```python
from build123d import *

# Parameters (mm, degrees)
SKETCH_1_R      = 2
EXTRUDE_1_DEPTH = 250


with BuildPart() as part:
    # 草图1 → 凸台-拉伸1 (new, symmetric)
    with BuildSketch(Plane.XY):
        with BuildLine():
            Line((-8.5, 0), (-3.95, 0))
            ThreePointArc((-3.95, 0), (-3.737867966, 0.087867966), (-3.65, 0.3))
            Line((-3.65, 0.3), (-3.65, 0.6))
            Line((-3.65, 0.6), (-3.1, 0.6))
            Line((-3.1, 0.6), (-3.1, 1.8))
            Line((-3.1, 1.8), (-5.6, 1.8))
            Line((-5.6, 1.8), (-5.6, 3.692893219))
            Line((-5.6, 3.692893219), (-3.192893219, 6.1))
            Line((-3.192893219, 6.1), (3.192893219, 6.1))
            Line((3.192893219, 6.1), (5.6, 3.692893219))
            Line((5.6, 3.692893219), (5.6, 1.8))
            Line((5.6, 1.8), (3.1, 1.8))
            Line((3.1, 1.8), (3.1, 0.6))
            Line((3.1, 0.6), (3.65, 0.6))
            Line((3.65, 0.6), (3.65, 0.3))
            ThreePointArc((3.65, 0.3), (3.737867966, 0.087867966), (3.95, 0))
            Line((3.95, 0), (8.5, 0))
            ThreePointArc((8.5, 0), (9.560660172, 0.439339828), (10, 1.5))
            Line((10, 1.5), (10, 8.5))
            ThreePointArc((10, 8.5), (9.560660172, 9.560660172), (8.5, 10))
            Line((8.5, 10), (-8.5, 10))
            ThreePointArc((-8.5, 10), (-9.560660172, 9.560660172), (-10, 8.5))
            Line((-10, 8.5), (-10, 1.5))
            ThreePointArc((-10, 1.5), (-9.560660172, 0.439339828), (-8.5, 0))
        make_face()
        with Locations((-7, 7)):
            Circle(SKETCH_1_R, mode=Mode.SUBTRACT)
        with Locations(Location((7, 7, 0), (0, 0, 180))):
            Circle(SKETCH_1_R, mode=Mode.SUBTRACT)
    extrude(amount=EXTRUDE_1_DEPTH, both=True)


solid = part.part
```
The model under review builds one solid part; all positions refer to its coordinate system, in mm. Round coordinates to 2 decimals unless told otherwise and drop trailing zeros. Order: outer loops, then holes, each group sorted by start corner. A loop starts at its lowest first (then second) coordinate and runs counter-clockwise, first axis right, second up. Notation, with made-up numbers: (60.25, 61.5) -> (119.25, 61.5) arc R6 cw to (119.25, 66.5) -> close; hole circle Ø8 at (73, -23.75). An arc over 180 degrees is marked (long way). Use a Markdown table: item, result.
Q1. Clearance check with flat-ended pins moving along their axes: P1, Ø2.5, axis at x = 7, y = 7, coming from the +Z side; P2, Ø0.6, axis at y = 1, z = -57.5, coming from the +X side. State where each tip first meets the part, or that it passes through.
Values:
| item | result |
|---|---|
| P1 | passes through |
| P2 | stops at x = 9.99 |
Q2. For line 1 (X direction, y = 7.5, z = 18); line 2 (X direction, y = 3.5, z = -157); line 3 (X direction, y = 1.5, z = 22), list the stretches that pass through material, from the lowest coordinate up.
Values:
| item | result |
|---|---|
| line 1 | x = -10 to -8.94, -5.06 to 5.06, 8.94 to 10 |
| line 2 | x = -10 to -5.6, 5.6 to 10 |
| line 3 | x = -10 to -3.1, 3.1 to 10 |
Q3. We need section A-A on z = 121. Write out the cut boundary in (x, y).
Values:
| item | result |
|---|---|
| outline | (-10, 1.5) arc R1.5 ccw to (-8.5, 0) -> (-3.95, 0) arc R0.3 ccw to (-3.65, 0.3) -> (-3.65, 0.6) -> (-3.1, 0.6) -> (-3.1, 1.8) -> (-5.6, 1.8) -> (-5.6, 3.69) -> (-3.19, 6.1) -> (3.19, 6.1) -> (5.6, 3.69) -> (5.6, 1.8) -> (3.1, 1.8) -> (3.1, 0.6) -> (3.65, 0.6) -> (3.65, 0.3) arc R0.3 ccw to (3.95, 0) -> (8.5, 0) arc R1.5 ccw to (10, 1.5) -> (10, 8.5) arc R1.5 ccw to (8.5, 10) -> (-8.5, 10) arc R1.5 ccw to (-10, 8.5) -> close; hole circle Ø4 at (-7, 7); hole circle Ø4 at (7, 7) |
